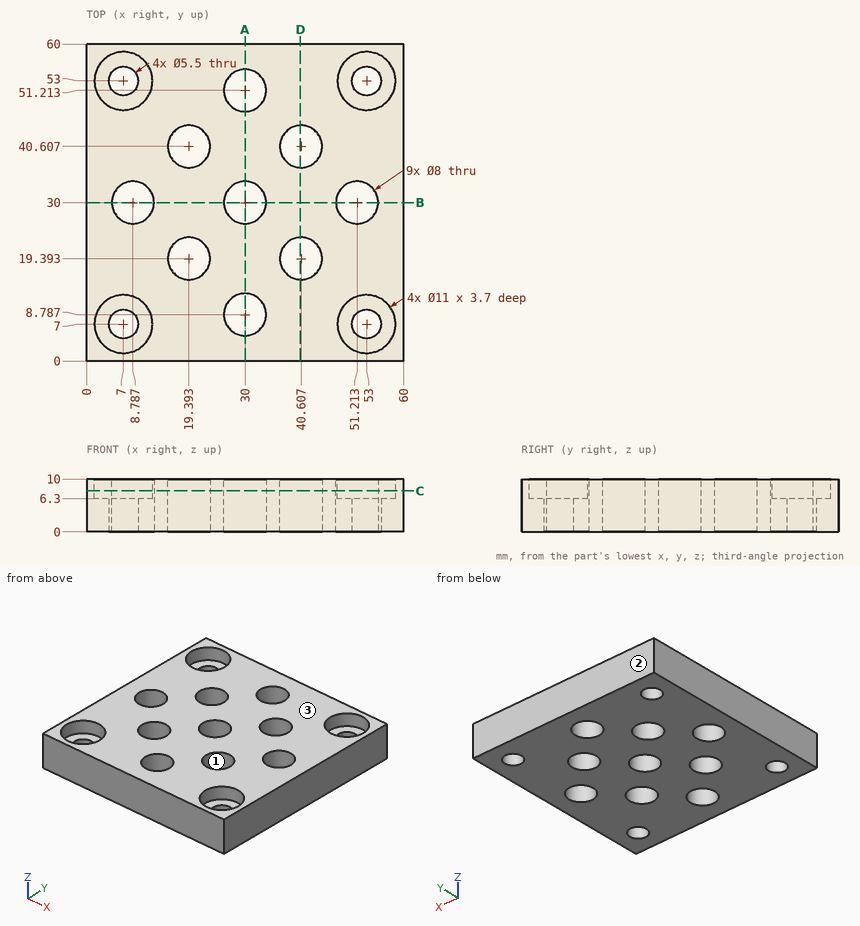
Geometry check sheet. Reference: drawing and pictorial views, mm from the part's lowest x, y, z. Round coordinates to 2 decimals unless told otherwise and drop trailing zeros. Write each loop counter-clockwise with the first axis right and the second up, starting at its lowest first coordinate (ties: lowest second). Pieces come first, ordered by that corner, then holes. Notation, with made-up numbers: (9, 58.25) -> (14, 58.25) arc R23 ccw to (14, 84.25) -> close; hole circle Ø7 at (-26.5, 5.5). An arc over 180 degrees is marked (long way). Put each result on its own line as item: value.
1) Cross-section at D-D, the plane x = 40.5. Enter the section's corners in (y, z) (1 decimal).
Recorded:
outline: (0, 0) -> (15.4, 0) -> (15.4, 10) -> (0, 10) -> close; (23.4, 0) -> (36.6, 0) -> (36.6, 10) -> (23.4, 10) -> close; (44.6, 0) -> (60, 0) -> (60, 10) -> (44.6, 10) -> close
2) Cross-section at C-C, the plane z = 7.75. Give the number of separate pieces and of enclosed holes in the cut face, plus the area to 3 significant figures.
Recorded:
separate pieces: 1
enclosed holes: 13
area: 2,770 mm2
3) Depth check by flat-ended pin: P1, Ø5.5, axis at x = 6, y = 7.5, coming from the +Z side. Enter the tip coordinate at first touch or a pass-through.
Recorded:
P1: stops at z = 6.3
4) Release check for a two-part mould opening along Y. For the marked faces 1, 2 and 3 record: pulls with the +Y half, pulls with the -Y half, needs draft (parallel to the pull), parting line crosses it, or undercut.
Recorded:
face 1: undercut
face 2: pulls with the +Y half
face 3: needs draft
5) Thickness scan on probe 1 along Y at (x, z) = (30, 5); probe 2 along Y at (x, z) = (49, 7.5) (1 decimal); probe 3 along X at (y, z) = (21.5, 0.75) (1 decimal). Record the ranges inside material, lowest first. Write a range as from..to.
Recorded:
probe 1: y = 0..4.79, 12.79..26, 34..47.21, 55.21..60
probe 2: y = 0..3.2, 10.8..26.7, 33.3..49.2, 56.8..60
probe 3: x = 0..16, 22.8..37.2, 44..60
6) Cross-section at A-A, the plane x = 30. Enter the section's corners in (y, z), plus the area to 3 significant figures.
Recorded:
outline: (0, 0) -> (4.79, 0) -> (4.79, 10) -> (0, 10) -> close; (12.79, 0) -> (26, 0) -> (26, 10) -> (12.79, 10) -> close; (34, 0) -> (47.21, 0) -> (47.21, 10) -> (34, 10) -> close; (55.21, 0) -> (60, 0) -> (60, 10) -> (55.21, 10) -> close
area: 360 mm2
